Print and shaded views of the part. All mm, measured from the part's lowest x, y and z. A direction names the side the tool comes from. Coordinates: 2 decimals unless noted, no trailing zeros. Loops run counter-clockwise (first coordinate to the right, second up) from the corner with the lowest first, then second, coordinate; pieces in that order, holes last. Notation, with made-up numbers: M 72.5,24 L 128.5,24 A15 cw 128.5,38 Z; hole C 64,29.5 d9. An arc over 180 degrees is marked long. Answer as a JSON object with one key per item and string values. Group by question number.
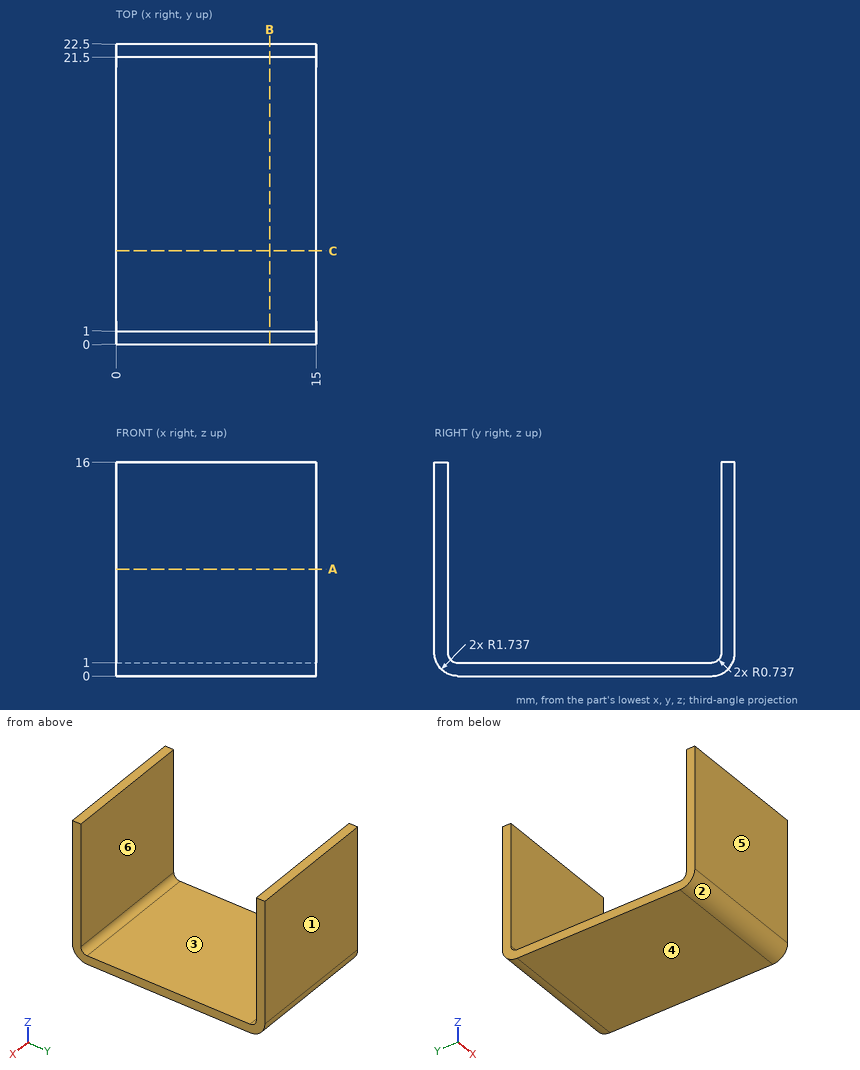
Item 1: Tool access for the marked faces 5 and 6: list every direction of +Z, -Z, +X, -X, +Y, -Y with a clear straight run to the whole face (end or side of a thin tool).
Item 2: Slice it at C-C, the plane y = 7. Write the cut outline in (x, z).
Item 3: Drill centre lines: L1, parallel to Y at x = 5.5, z = 12.5; L2, parallel to Z at x = 13.5, y = 6.75; L3, parallel to Z at x = 13, y = 21.75. Where is each one in solid material? Low to high. Write a range as from..to.
Item 4: Pull direction Y, two halves, no side cores. Call the marked faces 1, 2, 3 and 4: released by +Y, released by -Y, zero draft, split by the parting line, or undercut.
Item 5: Slice it at B-B, the plane x = 11.5. Write the cut outline in (y, z).
Item 6: Slice it at A-A, the plane z = 8. Write the cut outline in (x, y).
Item 7: Pin check, flat tips, straight feed: pin 1 (6 mm diameter, centred on y = 11.5, z = 6.5, fed in from +X) (3 decimals); pin 2 (1.5 mm diameter, centred on x = 10, y = 9, fed in from +Z). Stop position of each tip, or through.
Computed:
{
 "1": {"face 5": "+Z, -Z, +X, -X, -Y", "face 6": "+Z, +X, -X"},
 "2": {"outline": "M 0,0 L 15,0 L 15,1 L 0,1 Z"},
 "3": {"L1": "0..1, 21.5..22.5", "L2": "0..1", "L3": "0.31..16"},
 "4": {"face 1": "released by +Y", "face 2": "released by -Y", "face 3": "undercut", "face 4": "zero draft"},
 "5": {"outline": "M 0,1.74 A1.74 ccw 1.74,0 L 20.76,0 A1.74 ccw 22.5,1.74 L 22.5,16 L 21.5,16 L 21.5,1.74 A0.74 cw 20.76,1 L 1.74,1 A0.74 cw 1,1.74 L 1,16 L 0,16 Z"},
 "6": {"outline": "M 0,0 L 15,0 L 15,1 L 0,1 Z; M 0,21.5 L 15,21.5 L 15,22.5 L 0,22.5 Z"},
 "7": {"pin 1": "through", "pin 2": "z = 1"}
}
